```python
from build123d import *

# Parameters (mm, degrees)
SKETCH1_R           = 14
SKETCH1_R_2         = 13.15
BOSS_EXTRUDE1_DEPTH = 3
BOSS_EXTRUDE2_START = 1
SKETCH2_R           = 14
SKETCH2_R_2         = 9.025
BOSS_EXTRUDE2_DEPTH = 1
CUT_EXTRUDE1_DEPTH  = 21.055785441
CUT_EXTRUDE2_DEPTH  = 0.5


with BuildPart() as part:
    # Sketch1 → Boss-Extrude1 (new body)
    with BuildSketch(Plane.XY):
        with Locations((0.026824761, 0.017229283)):
            Circle(SKETCH1_R)
        with Locations((0.026824761, 0.017229283)):
            Circle(SKETCH1_R_2, mode=Mode.SUBTRACT)
    extrude(amount=-BOSS_EXTRUDE1_DEPTH)

    # Sketch2 → Boss-Extrude2 (add)
    with BuildSketch(Plane.XY.offset(BOSS_EXTRUDE2_START)):
        with Locations((0.026824761, 0.017229283)):
            Circle(SKETCH2_R)
        Circle(SKETCH2_R_2, mode=Mode.SUBTRACT)
    extrude(amount=-BOSS_EXTRUDE2_DEPTH)

    # Sketch3 → Cut-Extrude1 (cut, through all)
    with BuildSketch(Plane(origin=(0, 0, 0), x_dir=(-1, 0, 0), z_dir=(0, 0, -1))):
        with BuildLine():
            Line((-1.684865059, -13.02782351), (-0.026824761, -9.024960135))
            ThreePointArc((-0.026824761, -9.024960135), (-3.480481432, -8.326876605), (-6.403627708, -6.359573664))
            Line((-6.403627708, -6.359573664), (-6.420618215, -6.376564171))
            Line((-6.420618215, -6.376564171), (-8.078658513, -10.379427546))
            ThreePointArc((-8.078658513, -10.379427546), (-5.059111896, -12.131786569), (-1.684865059, -13.02782351))
        make_face()
    extrude(amount=-CUT_EXTRUDE1_DEPTH, mode=Mode.SUBTRACT)

    # Sketch4 → Cut-Extrude2 (cut)
    with BuildSketch(Plane.XY.offset(1)):
        with BuildLine():
            ThreePointArc((-6.362642541, 6.400578481), (-3.426918892, 8.349062936), (0.031150913, 9.024946239))
            Line((0.031150913, 9.024946239), (-1.640669197, 13.061077025))
            ThreePointArc((-1.640669197, 13.061077025), (-5.009864402, 12.164420822), (-8.025008992, 10.413886112))
            Line((-8.025008992, 10.413886112), (-6.362642541, 6.400578481))
        make_face()
    extrude(amount=-CUT_EXTRUDE2_DEPTH, mode=Mode.SUBTRACT)


solid = part.part
```
Here's how the part is built. I have some questions about the finished solid (model axes, mm). A direction names the side the tool comes from. Round coordinates to 2 decimals unless told otherwise and drop trailing zeros. Write each loop counter-clockwise with the first axis right and the second up, starting at its lowest first coordinate (ties: lowest second). Pieces come first, ordered by that corner, then holes.
Q1. Will these pins go through, and if not, where does the flat tip stop? P1, Ø1.5, axis at x = 4, z = -1.5, coming from the -Y side; P2, Ø1.5, axis at y = -6.5, z = 0, coming from the -X side; P3, Ø3.5, axis at x = -2, y = 8.5, coming from the +Z side.
Q2. If we mould it in two halves opening along X, with no side actions, what happens to faces 1 (the flat face through (-0.79, 11.01, 0.75)), 2 (the cylindrical face through (13.38, 4.22, -0.97)), 3 (the flat face through (9.2, 0.2, 1))? For each: +X half, -X half, draft (parallel to the pull), parting line (faces both ways), or undercut.
Q3. Please list where these lines run through material, in increasing order: probe 1 along Y at (x, z) = (0, 0.35) (3 decimals); probe 2 along X at (y, z) = (0, 0.4) (3 decimals); probe 3 along Z at (x, y) = (-11.5, -2).
Q4. If we section it at D-D on y = 4.25: Write out the boundary of the cut face in (x, z).
Q5. If we section it at C-C on z = -1.3: Write out the boundary of the cut face in (x, y).
Q6. If we section it at B-B on y = 8.5: Write out the boundary of the cut face in (x, z).
Q7. If we section it at A-A on x = -2.5: Write out the boundary of the cut face in (y, z), plus the area to 3 significant figures.
Q8. Which directions (+Z, -Z, +X, -X, +Y, -Y) give clear straight access to the entire face, cutting with the end or side of a thin tool? Please do faces 4 (the flat face through (4, 13, -3)), 5 (the flat face through (3, 9, 0)), 6 (the flat face through (0.867, -11.054, 0.493)), 7 (the flat face through (-4, 10, 0.5)).
Answer below:
1. P1: stops at y = -13.61
1. P2: stops at x = -12.73
1. P3: stops at z = 0.5
2. face 1: undercut
2. face 2: parting line
2. face 3: draft
3. probe 1: y = -13.983 to -9.025, 9.025 to 14.017
3. probe 2: x = -13.973 to -9.025, 9.025 to 14.027
3. probe 3: z = 0 to 1
4. outline: (-13.32, -3) - (-12.42, -3) - (-12.42, 0) - (-7.96, 0) - (-7.96, 1) - (-13.32, 1) - close; (7.96, 0) - (12.48, 0) - (12.48, -3) - (13.37, -3) - (13.37, 1) - (7.96, 1) - close
5. outline: circle Ø28 at (0.03, 0.02); hole circle Ø26.3 at (0.03, 0.02)
6. outline: (-11.11, -3) - (-10.02, -3) - (-10.02, 0) - (-3.03, 0) - (-3.03, 0.5) - (-7.23, 0.5) - (-7.23, 1) - (-11.11, 1) - close; (3.03, 0) - (10.07, 0) - (10.07, -3) - (11.16, -3) - (11.16, 1) - (3.03, 1) - close
7. outline: (-13.75, -3) - (-12.89, -3) - (-12.89, 0) - (-8.67, 0) - (-8.67, 1) - (-13.75, 1) - close; (8.67, 0) - (12.92, 0) - (12.92, -3) - (13.79, -3) - (13.79, 1) - (12.92, 1) - (12.92, 0.5) - (8.67, 0.5) - close
7. area: 13.3 mm2
8. face 4: -Z, +X, -X, +Y, -Y
8. face 5: -Z
8. face 6: +Z, -Z
8. face 7: +Z
